```python
from build123d import *

# Parameters (mm, degrees)
SKETCH_1_R          = 13.5
EXTRUDE_1_DEPTH     = 30
SKETCH_2_R          = 12
EXTRUDE_2_DEPTH     = 30
SKETCH_3_R          = 3
EXTRUDE_3_DEPTH     = 2
CUT_EXTRUDE_1_DEPTH = 5
SKETCH_5_R          = 1.25
EXTRUDE_4_DEPTH     = 5
FILLET_1_R          = 0.5


with BuildPart() as part:
    # 草图1 → 凸台-拉伸1 (new body)
    with BuildSketch(Plane.XY):
        Circle(SKETCH_1_R)
    extrude(amount=EXTRUDE_1_DEPTH)

    # 草图2 → 凸台-拉伸2 (add)
    with BuildSketch(Plane.XY.offset(30)):
        Circle(SKETCH_2_R)
    extrude(amount=EXTRUDE_2_DEPTH)

    # 草图3 → 凸台-拉伸3 (add)
    with BuildSketch(Plane.XY.offset(60)):
        Circle(SKETCH_3_R)
    extrude(amount=EXTRUDE_3_DEPTH)

    # 草图4 → 切除-拉伸1 (cut)
    with BuildSketch(Plane(origin=(0, 0, 0), x_dir=(-1, 0, 0), z_dir=(0, 0, -1))):
        with BuildLine():
            Line((-1, 12), (-1, 13.978745528))
            Line((-1, 13.978745528), (1, 13.978745528))
            Line((1, 13.978745528), (1, 12))
            ThreePointArc((1, 12), (0, 11), (-1, 12))
        make_face()
        with BuildLine():
            Line((10.892304845, -5.133974596), (12.60594874, -6.12334736))
            Line((12.60594874, -6.12334736), (11.60594874, -7.855398168))
            Line((11.60594874, -7.855398168), (9.892304845, -6.866025404))
            ThreePointArc((9.892304845, -6.866025404), (9.526279442, -5.5), (10.892304845, -5.133974596))
        make_face()
        with BuildLine():
            Line((-9.892304845, -6.866025404), (-11.60594874, -7.855398168))
            Line((-11.60594874, -7.855398168), (-12.60594874, -6.12334736))
            Line((-12.60594874, -6.12334736), (-10.892304845, -5.133974596))
            ThreePointArc((-10.892304845, -5.133974596), (-9.526279442, -5.5), (-9.892304845, -6.866025404))
        make_face()
    extrude(amount=-CUT_EXTRUDE_1_DEPTH, mode=Mode.SUBTRACT)

    # 草图5 → 凸台-拉伸4 (add)
    with BuildSketch(Plane(origin=(0, 0, 0), x_dir=(-1, 0, 0), z_dir=(0, 0, -1))):
        with Locations(Location((0, 0, 0), (0, 0, 180))):
            Circle(SKETCH_5_R)
        with Locations(Location((6, 0, 0), (0, 0, 180))):
            Circle(SKETCH_5_R)
    extrude(amount=EXTRUDE_4_DEPTH)

    # 圆角1
    fillet_1_edges = [part.edges().sort_by_distance(p)[0] for p in [
        (-1.25, 0, -5),
        (-7.25, 0, -5),
    ]]
    fillet(fillet_1_edges, radius=FILLET_1_R)


solid = part.part
```
Geometry: final body of the model. Coordinates: model frame, mm. A direction names the side the tool comes from. Round coordinates to 2 decimals unless told otherwise and drop trailing zeros. Loops run counter-clockwise (first coordinate to the right, second up) from the corner with the lowest first, then second, coordinate; pieces in that order, holes last. Notation, with made-up numbers: (42, 14) -> (78, 14) arc R29 cw to (78, 51) -> close; hole circle Ø1 at (-20, -5.75). An arc over 180 degrees is marked (long way). Use one line per item in the form item = value. Start each with the question number.
1) Access query for faces 4 (the cylindrical face through (-3, 0, 61)), 5 (the cylindrical face through (0, 11, 2)), 6 (the flat face through (11.53, -5.5, 2.46)). Directions: +Z, -Z, +X, -X, +Y, -Y. A direction counts if a zero-diameter tool reaches every point of the face in a straight line with its end or side. Return the directions, or none.
2) Section C-C on z = 39.5. Output: boundary loops of the cut face in (x, y).
3) Section B-B on y = 0. Output: boundary loops of the cut face in (x, z).
4) Draft query along X for faces 1 (the flat face through (1, 13, 2)), 2 (the flat face through (2.5, -2.5, 60)), 3 (the flat face through (-10.535, -7.237, 2.465)). Return one class per face: released by +X, released by -X, zero draft, split by the parting line, or undercut.
5) Section A-A on x = 0. Output: boundary loops of the cut face in (y, z).
6) Section D-D on y = -9.75. Output: boundary loops of the cut face in (x, z).
7) Line query: L1, parallel to Z at x = -10, y = -4.25; L2, parallel to Y at x = 5, z = 36; L3, parallel to Z at x = -0.5, y = 2. Output: solid intervals per line, ascending.
8) First-contact query: P1, Ø5, axis at x = 9, y = 5.5, coming from the -Z side; P2, Ø2, axis at x = 10, z = 17.5, coming from the +Y side; P3, Ø12, axis at x = -6.5, z = 30.5, coming from the +Y side. Flat tips, straight axial feed; report the tip coordinate or a pass-through.
Response:
q1.face_4 = +Z
q1.face_5 = -Z, +Y
q1.face_6 = -Z
q2.outline = circle Ø24 at (0, 0)
q3.outline = (-13.5, 0) -> (-7.25, 0) -> (-7.25, -4.5) arc R0.5 ccw to (-6.75, -5) -> (-5.25, -5) arc R0.5 ccw to (-4.75, -4.5) -> (-4.75, 0) -> (-1.25, 0) -> (-1.25, -4.5) arc R0.5 ccw to (-0.75, -5) -> (0.75, -5) arc R0.5 ccw to (1.25, -4.5) -> (1.25, 0) -> (13.5, 0) -> (13.5, 30) -> (12, 30) -> (12, 60) -> (3, 60) -> (3, 62) -> (-3, 62) -> (-3, 60) -> (-12, 60) -> (-12, 30) -> (-13.5, 30) -> close
q4.face_1 = undercut
q4.face_2 = zero draft
q4.face_3 = released by -X
q5.outline = (-13.5, 0) -> (-1.25, 0) -> (-1.25, -4.5) arc R0.5 ccw to (-0.75, -5) -> (0.75, -5) arc R0.5 ccw to (1.25, -4.5) -> (1.25, 0) -> (11, 0) -> (11, 5) -> (13.5, 5) -> (13.5, 30) -> (12, 30) -> (12, 60) -> (3, 60) -> (3, 62) -> (-3, 62) -> (-3, 60) -> (-12, 60) -> (-12, 30) -> (-13.5, 30) -> close
q6.outline = (-9.34, 0) -> (9.34, 0) -> (9.34, 30) -> (7, 30) -> (7, 60) -> (-7, 60) -> (-7, 30) -> (-9.34, 30) -> close
q7.L1 = 0 to 60
q7.L2 = -10.91 to 10.91
q7.L3 = 0 to 62
q8.P1 = 0
q8.P2 = 10.06
q8.P3 = 13.49
